For this review, take the finished solid that the model builds, in its own axes (mm). A direction names the side the tool comes from. Coordinates: 2 decimals unless noted, no trailing zeros. Loops run counter-clockwise (first coordinate to the right, second up) from the corner with the lowest first, then second, coordinate; pieces in that order, holes last. Notation, with made-up numbers: (-36.5, 38.5) -> (13.5, 38.5) arc R21 ccw to (13.5, 45.5) -> close; hole circle Ø6 at (77.5, -6.5). An arc over 180 degrees is marked (long way). One line per item, written item: value.
from build123d import *

# Parameters (mm, degrees)
CROQUIS1_W              = 108
CROQUIS1_H              = 26
SALIENTE_EXTRUIR2_DEPTH = 2
CROQUIS3_R              = 1.5
CORTAR_EXTRUIR3_DEPTH   = 10
CROQUIS5_W              = 108
CROQUIS5_H              = 26
CROQUIS5_R              = 1.5
SALIENTE_EXTRUIR4_DEPTH = 2
CROQUIS6_R              = 2.5
CORTAR_EXTRUIR4_DEPTH   = 2.25
CROQUIS7_W              = 108
CROQUIS7_H              = 26
CROQUIS7_W_2            = 106
CROQUIS7_H_2            = 24
CORTAR_EXTRUIR5_DEPTH   = 19


with BuildPart() as part:
    # Croquis1 → Saliente-Extruir2 (new body)
    with BuildSketch(Plane(origin=(0, 0, 0), x_dir=(1, 0, 0), z_dir=(0, 1, 0))):
        Rectangle(CROQUIS1_W, CROQUIS1_H)
    extrude(amount=SALIENTE_EXTRUIR2_DEPTH)

    # Croquis3 → Cortar-Extruir3 (cut)
    with BuildSketch(Plane(origin=(0, 2, 0), x_dir=(1, 0, 0), z_dir=(0, 1, 0))):
        with Locations(Location((-49, 8, 0), (0, 0, 270))):
            Circle(CROQUIS3_R)
        with Locations(Location((-49, -8, 0), (0, 0, 270))):
            Circle(CROQUIS3_R)
        with Locations(Location((49, -8, 0), (0, 0, 270))):
            Circle(CROQUIS3_R)
        with Locations(Location((49, 8, 0), (0, 0, 270))):
            Circle(CROQUIS3_R)
    extrude(amount=-CORTAR_EXTRUIR3_DEPTH, mode=Mode.SUBTRACT)

    # Croquis5 → Saliente-Extruir4 (add)
    with BuildSketch(Plane.XZ):
        Rectangle(CROQUIS5_W, CROQUIS5_H)
        with Locations(Location((-49, -8, 0), (0, 0, 90))):
            Circle(CROQUIS5_R, mode=Mode.SUBTRACT)
        with Locations(Location((-49, 8, 0), (0, 0, 90))):
            Circle(CROQUIS5_R, mode=Mode.SUBTRACT)
        with Locations(Location((49, 8, 0), (0, 0, 90))):
            Circle(CROQUIS5_R, mode=Mode.SUBTRACT)
        with Locations(Location((49, -8, 0), (0, 0, 90))):
            Circle(CROQUIS5_R, mode=Mode.SUBTRACT)
    extrude(amount=SALIENTE_EXTRUIR4_DEPTH)

    # Croquis6 → Cortar-Extruir4 (cut)
    with BuildSketch(Plane.XZ.offset(2)):
        with Locations(Location((-49, -8, 0), (0, 0, 270))):
            Circle(CROQUIS6_R)
        with Locations(Location((-49, 8, 0), (0, 0, 270))):
            Circle(CROQUIS6_R)
        with Locations(Location((49, -8, 0), (0, 0, 270))):
            Circle(CROQUIS6_R)
        with Locations(Location((49, 8, 0), (0, 0, 270))):
            Circle(CROQUIS6_R)
    extrude(amount=-CORTAR_EXTRUIR4_DEPTH, mode=Mode.SUBTRACT)

    # Croquis7 → Cortar-Extruir5 (cut)
    with BuildSketch(Plane.XZ.offset(2)):
        Rectangle(CROQUIS7_W, CROQUIS7_H)
        Rectangle(CROQUIS7_W_2, CROQUIS7_H_2, mode=Mode.SUBTRACT)
    extrude(amount=-CORTAR_EXTRUIR5_DEPTH, mode=Mode.SUBTRACT)


solid = part.part
1. The part is to be moulded in two halves that separate along Z. For faces 3 (the flat face through (-1, 0, -12)), 4 (the flat face through (-53, 0, 0)), 5 (the cylindrical face through (50.464, 1.137, -8.325)), say which applies: pulls with the +Z half, pulls with the -Z half, needs draft (parallel to the pull), parting line crosses it, or undercut.
Return value:
face 3: pulls with the -Z half
face 4: needs draft
face 5: undercut
2. Take a section at C-C, the plane x = -49. Give the boundary of the cut face in (y, z).
Return value:
outline: (-2, -12) -> (2, -12) -> (2, -9.5) -> (0.25, -9.5) -> (0.25, -10.5) -> (-2, -10.5) -> close; (-2, -5.5) -> (0.25, -5.5) -> (0.25, -6.5) -> (2, -6.5) -> (2, 6.5) -> (0.25, 6.5) -> (0.25, 5.5) -> (-2, 5.5) -> close; (-2, 10.5) -> (0.25, 10.5) -> (0.25, 9.5) -> (2, 9.5) -> (2, 12) -> (-2, 12) -> close
3. Take a section at A-A, the plane z = 8. Give the boundary of the cut face in (x, y), and give its area (3 significant figures).
Return value:
outline: (-53, -2) -> (-51.5, -2) -> (-51.5, 0.25) -> (-50.5, 0.25) -> (-50.5, 2) -> (-53, 2) -> close; (-47.5, 0.25) -> (-46.5, 0.25) -> (-46.5, -2) -> (46.5, -2) -> (46.5, 0.25) -> (47.5, 0.25) -> (47.5, 2) -> (-47.5, 2) -> close; (50.5, 0.25) -> (51.5, 0.25) -> (51.5, -2) -> (53, -2) -> (53, 2) -> (50.5, 2) -> close
area: 391 mm2
4. For faces 1 (the flat face through (47, 0.25, 8)), 2 (the cylindrical face through (-47.536, 1.137, -8.325)), list the 3-axis set-ups (+Z, -Z, +X, -X, +Y, -Y) from which the entire face can be reached by the end or side of a thin tool; tool diameter is ignored.
Return value:
face 1: -Y
face 2: +Y, -Y
5. Take a section at B-B, the plane y = -0.6. Give the boundary of the cut face in (x, z), and give its area (3 significant figures).
Return value:
outline: (-53, -12) -> (53, -12) -> (53, 12) -> (-53, 12) -> close; hole circle Ø5 at (-49, -8); hole circle Ø5 at (-49, 8); hole circle Ø5 at (49, -8); hole circle Ø5 at (49, 8)
area: 2,470 mm2
6. Insertion check: pin 1 Ø2.5 at (x, z) = (49, 8) entering from +Y; pin 2 Ø4.5 at (x, z) = (49, -8) entering from -Y. Each pin has a flat end and moves straight along its axis. Give the tip position at first contact, or say it passes through.
Return value:
pin 1: passes through
pin 2: stops at y = 0.25
7. To check wall thickness, follow probe 1 along X at (y, z) = (-1.2, -8); probe 2 along X at (y, z) = (1.1, 8); probe 3 along Z at (x, y) = (47.5, -0.65). State the ranges of each line that lie inside material, in increasing order. Write a range as from..to.
Return value:
probe 1: x = -53..-51.5, -46.5..46.5, 51.5..53
probe 2: x = -53..-50.5, -47.5..47.5, 50.5..53
probe 3: z = -12..-10, -6..6, 10..12
